Study the drawing (mm; zero at the part's minimum x, y, z) and answer. Coordinates: 2 decimals unless noted, no trailing zeros. Order: outer loops, then holes, each group sorted by start corner. A loop starts at its lowest first (then second) coordinate and runs counter-clockwise, first axis right, second up.
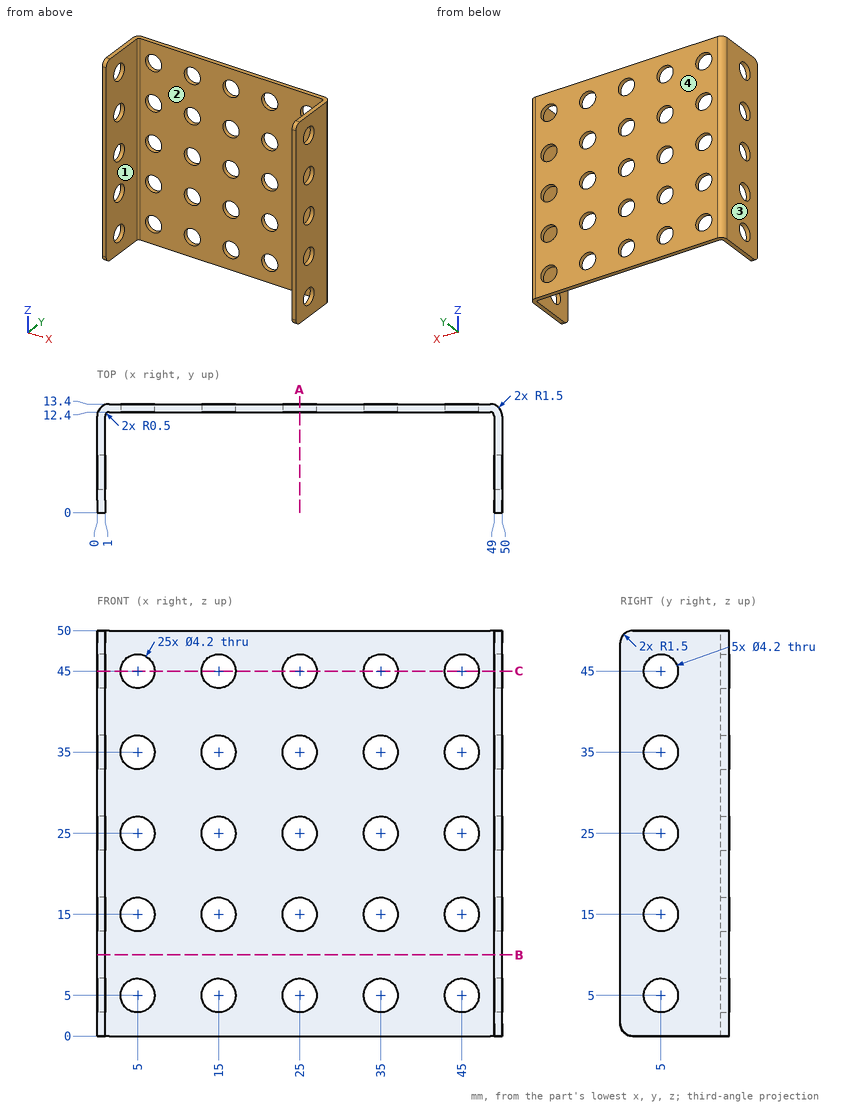
(1) Find section C-C (z = 45). Give the number of separate pieces and of enclosed holes in the cut face, and give its area (3 significant figures).
(2) Consider line 1 (Z direction, x = 49.35, y = 5); line 2 (X direction, y = 3.75, z = 11); line 3 (Y direction, x = 22, z = 30.5). Determine where each line is inside the solid, lowest interval first.
(3) Find section B-B (z = 10). Write down the section's boundary in (x, y), and give its area (3 significant figures).
(4) The mould has two halves that part along X. Classify the marked faces 1, 2, 3 and 4: released by +X, released by -X, zero draft, split by the parting line, or undercut.
(5) This flat-tipped pin is pushed along its axis until it touches: pin 1 Ø3 at (x, z) = (43.5, 28.5) entering from -Y. Where does it stop, or does it pass through?
(6) Find section A-A (x = 25). Write down the section's boundary in (y, z), and give its area (3 significant figures).
Findings below:
1. separate pieces: 8
1. enclosed holes: 0
1. area: 44.5 mm2
2. line 1: z = 0 to 2.9, 7.1 to 12.9, 17.1 to 22.9, 27.1 to 32.9, 37.1 to 42.9, 47.1 to 50
2. line 2: x = 0 to 1, 49 to 50
2. line 3: y = 12.4 to 13.4
3. outline: (0, 0) - (1, 0) - (1, 11.9) arc R0.5 cw to (1.5, 12.4) - (48.5, 12.4) arc R0.5 cw to (49, 11.9) - (49, 0) - (50, 0) - (50, 11.9) arc R1.5 ccw to (48.5, 13.4) - (1.5, 13.4) arc R1.5 ccw to (0, 11.9) - close
3. area: 73.9 mm2
4. face 1: undercut
4. face 2: undercut
4. face 3: released by -X
4. face 4: zero draft
5. pin 1: stops at y = 12.4
6. outline: (12.4, 0) - (13.4, 0) - (13.4, 2.9) - (12.4, 2.9) - close; (12.4, 7.1) - (13.4, 7.1) - (13.4, 12.9) - (12.4, 12.9) - close; (12.4, 17.1) - (13.4, 17.1) - (13.4, 22.9) - (12.4, 22.9) - close; (12.4, 27.1) - (13.4, 27.1) - (13.4, 32.9) - (12.4, 32.9) - close; (12.4, 37.1) - (13.4, 37.1) - (13.4, 42.9) - (12.4, 42.9) - close; (12.4, 47.1) - (13.4, 47.1) - (13.4, 50) - (12.4, 50) - close
6. area: 29.0 mm2
